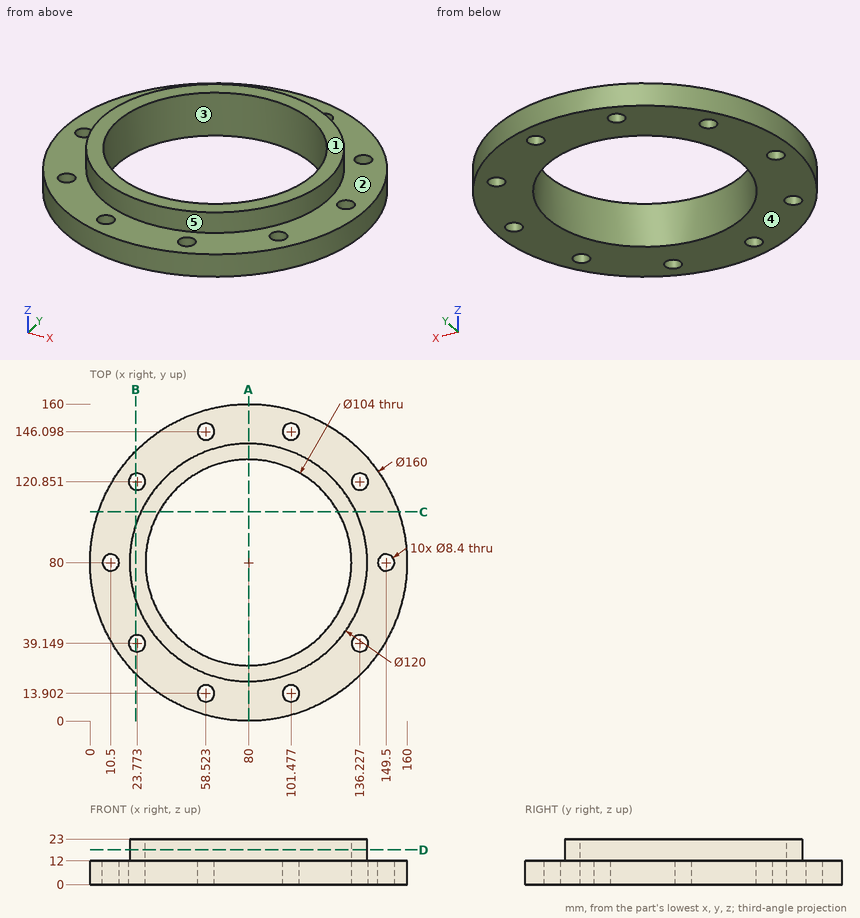
Check sheet for the drawn part. Datum: minimum x, y, z corner. Units: mm. A direction names the side the tool comes from. Round coordinates to 2 decimals unless told otherwise and drop trailing zeros. Write each loop counter-clockwise with the first axis right and the second up, starting at its lowest first coordinate (ties: lowest second). Pieces come first, ordered by that corner, then holes. Notation, with made-up numbers: (4.5, 58) - (60.5, 58) arc R22 cw to (60.5, 88) - close; hole circle Ø9 at (-17, 52.5). An arc over 180 degrees is marked (long way). Return JSON: item names as keys, results as strings.
Q1. Depth check by flat-ended pin: P1, Ø13.5, axis at x = 23.77, y = 120.85, coming from the +Z side; P2, Ø4, axis at x = 143.5, z = 20.5, coming from the +Y side; P3, Ø4, axis at y = 44, z = 16, coming from the -X side; P4, Ø1.5, axis at x = 142, z = 4.5, coming from the -Y side. Enter the tip coordinate at first touch or a pass-through.
Returned:
{"P1": "stops at z = 12", "P2": "passes through", "P3": "stops at x = 30.56", "P4": "stops at y = 28.54"}
Q2. Cross-section at C-C (y = 105.5). Record the boundary of the cut face in (x, z).
Returned:
{"outline": "(4.17, 0) - (34.68, 0) - (34.68, 23) - (25.69, 23) - (25.69, 12) - (4.17, 12) - close; (125.32, 0) - (155.83, 0) - (155.83, 12) - (134.31, 12) - (134.31, 23) - (125.32, 23) - close"}
Q3. Draft check along Y on the marked faces 3, 4 and 5. Enter one of: released by +Y, released by -Y, zero draft, split by the parting line, or undercut.
Returned:
{"face 3": "undercut", "face 4": "zero draft", "face 5": "split by the parting line"}
Q4. Cross-section at B-B (x = 23). Record the boundary of the cut face in (y, z) (1 decimal).
Returned:
{"outline": "(23.9, 0) - (35, 0) - (35, 12) - (23.9, 12) - close; (43.3, 0) - (116.7, 0) - (116.7, 12) - (98.7, 12) - (98.7, 23) - (61.3, 23) - (61.3, 12) - (43.3, 12) - close; (125, 0) - (136.1, 0) - (136.1, 12) - (125, 12) - close"}
Q5. Access from +Z, -Z, +X, -X, +Y, -Y to the whole of each face (thin tool, end or side, straight path). Record for the marked faces 1 and 2.
Returned:
{"face 1": "+Z, +X, -X, +Y, -Y", "face 2": "+Z"}
Q6. Scan lines: L1, parallel to Y at x = 133, z = 11.75 (1 decimal); L2, parallel to Z at x = 14.5, y = 59; L3, parallel to X at y = 13.5, z = 5 (1 decimal). Record each from-to range of solid material in increasing order. Write a range as from..to.
Returned:
{"L1": "y = 20.1..36.5, 41.8..118.2, 123.5..139.9", "L2": "z = 0..12", "L3": "x = 35.5..54.3, 62.7..97.3, 105.7..124.5"}
Q7. Cross-section at A-A (x = 80). Record the boundary of the cut face in (y, z), then the cut area to 3 significant figures.
Returned:
{"outline": "(0, 0) - (28, 0) - (28, 23) - (20, 23) - (20, 12) - (0, 12) - close; (132, 0) - (160, 0) - (160, 12) - (140, 12) - (140, 23) - (132, 23) - close", "area": "848 mm²"}
Q8. Cross-section at D-D (z = 17.5). Record the boundary of the cut face in (x, y).
Returned:
{"outline": "circle Ø120 at (80, 80); hole circle Ø104 at (80, 80)"}
